Can you work these out from the model? Positions are in its coordinate system, mm. Coordinates: 2 decimals unless noted, no trailing zeros. Write each loop counter-clockwise with the first axis right and the second up, starting at its lowest first coordinate (ties: lowest second). Pieces come first, ordered by that corner, then holes. Notation, with made-up numbers: (22.25, -17.75) - (65.25, -17.75) arc R16 ccw to (65.25, 3.25) - close; hole circle Ø3 at (48, -18). An arc over 180 degrees is marked (long way). One line per question, with ' | ' between items. Start each with the question number.
from build123d import *

# Parameters (mm, degrees)
F0_W     = 17
F0_H     = 8
F1_DEPTH = 50
F2_R     = 1.75
F3_DEPTH = 2.1
F4_R     = 1


with BuildPart() as f1:
    # F0 (on Top) → F1 (new body)
    with BuildSketch(Plane.XY):
        Rectangle(F0_W, F0_H)
    extrude(amount=F1_DEPTH)

    # F2 (on face) → F3 (join)
    with BuildSketch(Plane(origin=(0, 0, 0), x_dir=(1, 0, 0), z_dir=(0, 0, -1))):
        Circle(F2_R)
    extrude(amount=F3_DEPTH)

    # F4
    f4_edges = [f1.edges().sort_by_distance(p)[0] for p in [
        (-8.5, 4, 25),
        (8.5, 4, 25),
        (8.5, -4, 25),
        (-8.5, -4, 25),
    ]]
    fillet(f4_edges, radius=F4_R)


solid = f1.part
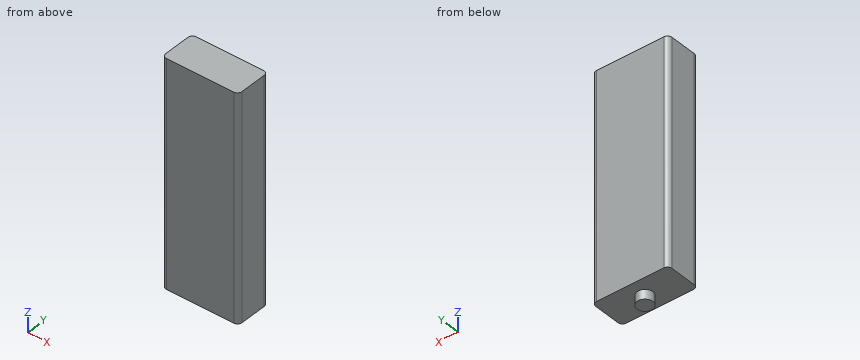
(1) If I drill on probe 1 along Z at (x, y) = (1.25, 2.75), over which ranges is the centre line in solid material (lowest first)?
(2) If we section it at D-D on x = -2.5: List the corners of the cut face in (y, z) for me, plus the area to 3 significant figures.
(3) If we section it at C-C on y = 2.25: List the corners of the cut face in (x, z) for me, plus the area to 3 significant figures.
(4) I'm going to push a flat-ended pin straight in: pin 1 (3 mm diameter, centred on x = -3, y = 3, fed in from -Z). Where does the tip first touch, or does it pass through?
(5) If we section it at A-A on y = 0: List the corners of the cut face in (x, z) for me.
(6) If we section it at B-B on x = 0: List the corners of the cut face in (y, z) for me, plus the area to 3 significant figures.
Values:
1) probe 1: 0 to 50
2) outline: (-4, 0) - (4, 0) - (4, 50) - (-4, 50) - close | area: 400 mm2
3) outline: (-8.5, 0) - (8.5, 0) - (8.5, 50) - (-8.5, 50) - close | area: 850 mm2
4) pin 1: z = 0
5) outline: (-8.5, 0) - (-1.75, 0) - (-1.75, -2.1) - (1.75, -2.1) - (1.75, 0) - (8.5, 0) - (8.5, 50) - (-8.5, 50) - close
6) outline: (-4, 0) - (-1.75, 0) - (-1.75, -2.1) - (1.75, -2.1) - (1.75, 0) - (4, 0) - (4, 50) - (-4, 50) - close | area: 407 mm2
